Geometry: final body of the model. Coordinates: model frame, mm. A direction names the side the tool comes from. Round coordinates to 2 decimals unless told otherwise and drop trailing zeros. Loops run counter-clockwise (first coordinate to the right, second up) from the corner with the lowest first, then second, coordinate; pieces in that order, holes last. Notation, with made-up numbers: (37.25, 1.25) - (44.25, 1.25) arc R22 ccw to (44.25, 32.25) - close; hole circle Ø8 at (-17, -23.75). An arc over 180 degrees is marked (long way). Answer in a Markdown table with one row per item. Add a question column.
from build123d import *

# Parameters (mm, degrees)
SKETCH4_W                 = 304.8
SKETCH4_H                 = 254
BOSS_EXTRUDE1_DEPTH       = 76.2
SKETCH5_W                 = 228.6
SKETCH5_H                 = 177.8
CUT_EXTRUDE1_DEPTH        = 38.1
FILLET1_R                 = 12.7
SKETCH11_W                = 12.7
SKETCH11_H                = 38.1
BOSS_EXTRUDE2_DEPTH       = 38.735
SKETCH12_R                = 9.525
CUT_EXTRUDE4_DEPTH        = 267.7
FILLET3_R                 = 6.35
SKETCH13_W                = 254
SKETCH13_H                = 3.81
CUT_EXTRUDE5_DEPTH        = 23.495
BOSS_EXTRUDE3_DEPTH       = 12.7
FILLET5_R                 = 6.35
F_8_32_TAPPED_HOLE1_D     = 3.4544
F_8_32_TAPPED_HOLE1_DEPTH = 9.652
F_8_32_TAPPED_HOLE1_TIP   = 1.037806461


with BuildPart() as part:
    # Sketch4 → Boss-Extrude1 (new body)
    with BuildSketch(Plane(origin=(0, 0, 0), x_dir=(1, 0, 0), z_dir=(0, 1, 0))):
        Rectangle(SKETCH4_W, SKETCH4_H)
    extrude(amount=BOSS_EXTRUDE1_DEPTH)

    # Sketch5 → Cut-Extrude1 (cut)
    with BuildSketch(Plane(origin=(0, 76.2, 0), x_dir=(1, 0, 0), z_dir=(0, 1, 0))):
        Rectangle(SKETCH5_W, SKETCH5_H)
    extrude(amount=-CUT_EXTRUDE1_DEPTH, mode=Mode.SUBTRACT)

    # Fillet1
    fillet1_edges = [part.edges().sort_by_distance(p)[0] for p in [
        (0, 0, 127),
        (-152.4, 0, 0),
        (0, 0, -127),
        (152.4, 0, 0),
        (152.4, 38.1, 127),
        (-152.4, 38.1, 127),
        (-152.4, 38.1, -127),
        (152.4, 38.1, -127),
    ]]
    fillet(fillet1_edges, radius=FILLET1_R)

    # Sketch11 → Boss-Extrude2 (add, symmetric)
    with BuildSketch(Plane(origin=(0, 76.2, 0), x_dir=(1, 0, 0), z_dir=(0, 1, 0))):
        with Locations((-107.95, 146.05)):
            Rectangle(SKETCH11_W, SKETCH11_H)
        with Locations((107.95, 146.05)):
            Rectangle(SKETCH11_W, SKETCH11_H)
    extrude(amount=BOSS_EXTRUDE2_DEPTH, both=True)

    # Sketch12 → Cut-Extrude4 (cut, through all)
    with BuildSketch(Plane.ZY.offset(114.3)):
        with Locations((-146.05, 101.6)):
            Circle(SKETCH12_R)
    extrude(amount=-CUT_EXTRUDE4_DEPTH, mode=Mode.SUBTRACT)

    # Fillet3
    fillet3_edges = [part.edges().sort_by_distance(p)[0] for p in [
        (-107.95, 114.935, -127),
        (107.95, 114.935, -127),
    ]]
    fillet(fillet3_edges, radius=FILLET3_R)

    # Sketch13 → Cut-Extrude5 (cut)
    with BuildSketch(Plane(origin=(0, 76.2, 0), x_dir=(1, 0, 0), z_dir=(0, 1, 0))):
        Rectangle(SKETCH13_W, SKETCH13_H)
    extrude(amount=-CUT_EXTRUDE5_DEPTH, mode=Mode.SUBTRACT)

    # Sketch18 → Boss-Extrude3 (add)
    with BuildSketch(Plane(origin=(-127, 0, 0), x_dir=(0, 0, -1), z_dir=(1, 0, 0))):
        with BuildLine():
            Line((-1.905, 52.705), (1.3e-08, 52.705))
            ThreePointArc((1.3e-08, 52.705), (-1.347038413, 53.262961577), (-1.905, 54.61))
            Line((-1.905, 54.61), (-1.905, 52.705))
        make_face()
        with BuildLine():
            Line((1.905, 52.705), (1.905, 54.61))
            ThreePointArc((1.905, 54.61), (1.347038423, 53.262961587), (1.3e-08, 52.705))
            Line((1.3e-08, 52.705), (1.905, 52.705))
        make_face()
    boss_extrude3 = extrude(amount=BOSS_EXTRUDE3_DEPTH)

    # Mirror1: Boss-Extrude3 across plane
    add(boss_extrude3.mirror(Plane(origin=(0, 0, 0), x_dir=(0, 0, 1), z_dir=(1, 0, 0))))

    # Fillet5
    fillet5_edges = [part.edges().sort_by_distance(p)[0] for p in [
        (-107.95, 37.465, -165.1),
        (-107.95, 114.935, -165.1),
        (107.95, 37.465, -165.1),
        (107.95, 114.935, -165.1),
    ]]
    fillet(fillet5_edges, radius=FILLET5_R)

    # #8-32 Tapped Hole1
    with Locations(Plane(origin=(0, 76.2, 0), x_dir=(1, 0, 0), z_dir=(0, 1, 0))):
        with Locations((-139.7, -114.3), (-139.7, 114.3), (139.7, 114.3), (139.7, -114.3)):
            Hole(F_8_32_TAPPED_HOLE1_D / 2, depth=F_8_32_TAPPED_HOLE1_DEPTH)
            with Locations((0, 0, -(F_8_32_TAPPED_HOLE1_DEPTH + F_8_32_TAPPED_HOLE1_TIP / 2))):  # 118° drill point
                Cone(0, F_8_32_TAPPED_HOLE1_D / 2, F_8_32_TAPPED_HOLE1_TIP, mode=Mode.SUBTRACT)


solid = part.part
1) Section A-A, the plane y = 101.6. Return the cut outline in (x, z) (3 decimals).
2) Contact query for flat-ended pins moving along their axis: pin 1 Ø8 at (x, y) = (77, 66) entering from -Z; pin 2 Ø19 at (y, z) = (77.5, -148) entering from -X; pin 3 Ø10 at (x, z) = (-107.5, -136.5) entering from -Y (3 decimals). Output: stop coordinate, or through.
3) Pull-direction query (X, two-part tool) for faces 5 (the flat face through (121, 66, -1.905)), 6 (the cylindrical face through (148.58, 3.62, -1.6)), 7 (the cylindrical face through (-108.04, 109.63, -140.93)); classes: pulls with the +X half, pulls with the -X half, needs draft (parallel to the pull), parting line crosses it, or undercut.
4) Section D-D, the plane x = -1. Return the cut outline in (y, z).
5) Section C-C, the plane x = -108. Return the cut outline in (y, z) (3 decimals).
6) Section B-B, the plane z = -146.05. Return the cut outline in (x, y) (3 decimals).
7) Material intervals for line 1 along X through (y, z) = (69, -114); line 2 along Z through (x, y) = (-29.5, 62.5); line 3 along X through (y, z) = (53, -62.5), sorted ascending. Write a range as from..to.
8) Reachability of faces 1 (the flat face through (-108, 37.465, -143)), 2 (the flat face through (-101.6, 76, -146)), 3 (the flat face through (108, 93, -127)), 4 (the flat face through (-2, 57, 88.9)) from +Z, -Z, +X, -X, +Y, -Y: full face, straight path, thin tool, end or side. Return the list, or none.
Evaluation:
| question | item | result |
|---|---|---|
| 1 | outline | (-114.3, -165.1) - (-101.6, -165.1) - (-101.6, -155.575) - (-114.3, -155.575) - close; (-114.3, -136.525) - (-101.6, -136.525) - (-101.6, -127) - (-114.3, -127) - close; (101.6, -165.1) - (114.3, -165.1) - (114.3, -155.575) - (101.6, -155.575) - close; (101.6, -136.525) - (114.3, -136.525) - (114.3, -127) - (101.6, -127) - close |
| 2 | pin 1 | stops at z = -127 |
| 2 | pin 2 | stops at x = -114.3 |
| 2 | pin 3 | stops at y = 37.465 |
| 3 | face 5 | undercut |
| 3 | face 6 | pulls with the +X half |
| 3 | face 7 | needs draft |
| 4 | outline | (0, -114.3) arc R12.7 ccw to (12.7, -127) - (76.2, -127) - (76.2, -88.9) - (38.1, -88.9) - (38.1, 88.9) - (76.2, 88.9) - (76.2, 127) - (12.7, 127) arc R12.7 ccw to (0, 114.3) - close |
| 5 | outline | (0, -114.3) arc R12.7 ccw to (12.7, -127) - (37.465, -127) - (37.465, -158.75) arc R6.35 ccw to (43.815, -165.1) - (108.585, -165.1) arc R6.35 ccw to (114.935, -158.75) - (114.935, -133.35) arc R6.35 ccw to (108.585, -127) - (76.2, -127) - (76.2, -88.9) - (38.1, -88.9) - (38.1, 88.9) - (76.2, 88.9) - (76.2, 127) - (12.7, 127) arc R12.7 ccw to (0, 114.3) - close; hole circle Ø19.05 at (101.6, -146.05) |
| 6 | outline | (-114.3, 37.465) - (-101.6, 37.465) - (-101.6, 92.075) - (-114.3, 92.075) - close; (-114.3, 111.125) - (-101.6, 111.125) - (-101.6, 114.935) - (-114.3, 114.935) - close; (101.6, 37.465) - (114.3, 37.465) - (114.3, 92.075) - (101.6, 92.075) - close; (101.6, 111.125) - (114.3, 111.125) - (114.3, 114.935) - (101.6, 114.935) - close |
| 7 | line 1 | x = -152.4..-141.4, -138..138, 141.4..152.4 |
| 7 | line 2 | z = -127..-88.9, 88.9..127 |
| 7 | line 3 | x = -152.4..-114.3, 114.3..152.4 |
| 8 | face 1 | -Z, +X, -X, -Y |
| 8 | face 2 | -Z, +Y, -Y |
| 8 | face 3 | +Z, +X, -X, +Y |
| 8 | face 4 | +Y |
